For this review, take the finished solid that the model builds, in its own axes (mm). Coordinates: 2 decimals unless noted, no trailing zeros. Order: outer loops, then holes, each group sorted by start corner. A loop starts at its lowest first (then second) coordinate and runs counter-clockwise, first axis right, second up. Notation, with made-up numbers: (20, 81) -> (66, 81) arc R14 ccw to (66, 99) -> close; hole circle Ø11 at (68, 88). An arc over 180 degrees is marked (long way). Write item = value, one per line. Start each with the question number.
1) Consider section B-B on y = -6. Give the boundary of the cut face in (x, z).
2) Wall thickness on probe 1 along Y at (x, z) = (3.5, 23); probe 2 along Z at (x, y) = (4.25, -6.75); probe 3 along Z at (x, y) = (8.5, -6): over which ranges is each line inside the solid? List them lowest first. Write a range as [from, to].
3) Consider section A-A on x = 6. Give the boundary of the cut face in (y, z).
4) Consider section D-D on y = -2.75. Give the boundary of the cut face in (x, z), and give its area (3 significant figures).
5) Consider section C-C on z = 46.5. Give the boundary of the cut face in (x, y).
6) Insertion check: pin 1 Ø3.5 at (x, z) = (7, 24.5) entering from -Y; pin 2 Ø1.5 at (y, z) = (-6.5, 36.5) entering from +X. Each pin has a flat end and moves straight along its axis. Give the tip position at first contact, or say it passes through.
from build123d import *

# Parameters (mm, degrees)
F1_DEPTH = 5
F2_R     = 3
F3_DEPTH = 3


with BuildPart() as f1:
    # F0 (on Front) → F1 (new body)
    with BuildSketch(Plane.XZ):
        with BuildLine():
            Line((0, 46), (0, 0))
            ThreePointArc((0, 0), (6, -6), (12, 0))
            Line((12, 0), (12, 46))
            ThreePointArc((12, 46), (6, 52), (0, 46))
        make_face()
    extrude(amount=F1_DEPTH)

    # F2 (on face) → F3 (join)
    with BuildSketch(Plane.XZ.offset(5)):
        with Locations((6, 46)):
            Circle(F2_R)
        with Locations((6, 0)):
            Circle(F2_R)
    extrude(amount=F3_DEPTH)


solid = f1.part
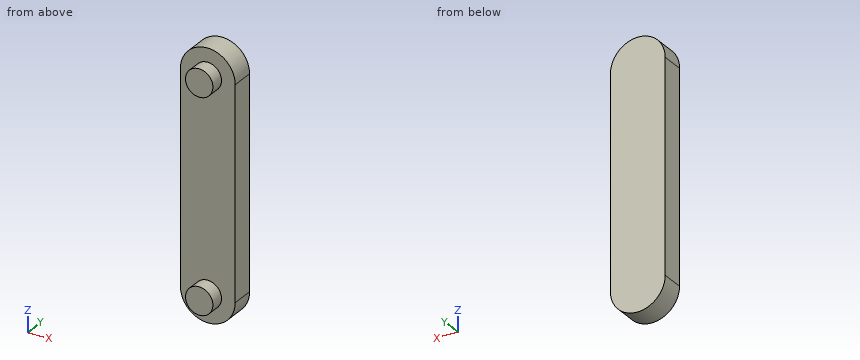
Answer sheet:
q1.outline = circle Ø6 at (6, 0); circle Ø6 at (6, 46)
q2.probe_1 = [-5, 0]
q2.probe_2 = [-2.44, 2.44], [43.56, 48.44]
q2.probe_3 = [-1.66, 1.66], [44.34, 47.66]
q3.outline = (-8, -3) -> (-5, -3) -> (-5, -6) -> (0, -6) -> (0, 52) -> (-5, 52) -> (-5, 49) -> (-8, 49) -> (-8, 43) -> (-5, 43) -> (-5, 3) -> (-8, 3) -> close
q4.outline = (0, 0) arc R6 ccw to (12, 0) -> (12, 46) arc R6 ccw to (0, 46) -> close
q4.area = 665 mm2
q5.outline = (0.02, -5) -> (3.04, -5) -> (3.04, -8) -> (8.96, -8) -> (8.96, -5) -> (11.98, -5) -> (11.98, 0) -> (0.02, 0) -> close
q6.pin_1 = -5
q6.pin_2 = through
